from build123d import *

# Parameters (mm, degrees)
BOSS_EXTRUDE1_DEPTH                           = 10
CBORE_FOR_M3_HEX_HEAD_MACHINE_SCREW3_AT_COUNT = 2
CBORE_FOR_M3_HEX_HEAD_MACHINE_SCREW3_AT_PITCH = 31.112698372
CBORE_FOR_M3_HEX_HEAD_MACHINE_SCREW3_2_COUNT  = 2
CBORE_FOR_M3_HEX_HEAD_MACHINE_SCREW3_2_PITCH  = 44
CUT_EXTRUDE1_START                            = -10
CUT_EXTRUDE1_DEPTH                            = 10


with BuildPart() as part:
    # Sketch1 → Boss-Extrude1 (new body)
    with BuildSketch(Plane.XY):
        with BuildLine():
            Line((-2.236067977, -2), (-21, -2))
            Line((-21, -2), (-21, 2))
            Line((-21, 2), (-2.236067977, 2))
            ThreePointArc((-2.236067977, 2), (0, 3), (2.236067977, 2))
            Line((2.236067977, 2), (24.919871589, 2))
            ThreePointArc((24.919871589, 2), (-25, 0), (24.919871589, -2))
            Line((24.919871589, -2), (2.236067977, -2))
            ThreePointArc((2.236067977, -2), (0, -3), (-2.236067977, -2))
        make_face()
    extrude(amount=BOSS_EXTRUDE1_DEPTH)

    # Sketch6 → CBORE for M3 Hex Head Machine Screw2 (revolve, cut)
    with BuildSketch(Plane(origin=(19.919871589, 22, 5), x_dir=(0, 0, 1), z_dir=(1, 0, 0))):
        Polygon((0, 0), (0, 47), (1.7, 47), (1.7, 17.3), (4.2, 17.3), (4.2, 0.025), (4.225, 0), align=None)
    revolve(axis=Axis((19.919871589, 28.35, 5), (0, -1, 0)), mode=Mode.SUBTRACT)

    # Sketch8 → CBORE for M3 Hex Head Machine Screw3 (revolve, cut)
    with BuildSketch(Plane(origin=(-15.556349186, 15.556349186, 10), x_dir=(0, -1, 0), z_dir=(1, 0, 0))):
        Polygon((0, 0), (0, 10), (1.7, 10), (1.7, 2.3), (4.2, 2.3), (4.2, 0.025), (4.225, 0), align=None)
    cbore_for_m3_hex_head_machine_screw3 = revolve(axis=Axis((-15.556349186, 15.556349186, 16.35), (0, 0, -1)), mode=Mode.SUBTRACT)

    # CBORE for M3 Hex Head Machine Screw3 at: CBORE for M3 Hex Head Machine Screw3 ×2
    with Locations(*[(0, -i * CBORE_FOR_M3_HEX_HEAD_MACHINE_SCREW3_AT_PITCH, 0) for i in range(1, CBORE_FOR_M3_HEX_HEAD_MACHINE_SCREW3_AT_COUNT)]):
        add(cbore_for_m3_hex_head_machine_screw3, mode=Mode.SUBTRACT)

    # CBORE for M3 Hex Head Machine Screw3 2: CBORE for M3 Hex Head Machine Screw3 ×2
    with Locations(*[Vector(0.707106781, -0.707106781, 0) * (i * CBORE_FOR_M3_HEX_HEAD_MACHINE_SCREW3_2_PITCH) for i in range(1, CBORE_FOR_M3_HEX_HEAD_MACHINE_SCREW3_2_COUNT)]):
        add(cbore_for_m3_hex_head_machine_screw3, mode=Mode.SUBTRACT)

    # Sketch9 → Cut-Extrude1 (cut)
    with BuildSketch(Plane(origin=(0, 0, 0), x_dir=(-1, 0, 0), z_dir=(0, 0, -1)).offset(CUT_EXTRUDE1_START)):
        with BuildLine():
            ThreePointArc((-17.370952766, 13.5), (-19.8577472, 9.46941794), (-21.424285286, 5))
            Line((-21.424285286, 5), (21.424285286, 5))
            ThreePointArc((21.424285286, 5), (20.018217875, 9.125291947), (17.826515683, 12.892452777))
            ThreePointArc((17.826515683, 12.892452777), (15.142522709, 12.080899913), (12.724136619, 13.5))
            Line((12.724136619, 13.5), (-17.370952766, 13.5))
        make_face()
        with BuildLine():
            Line((21.424285286, -5), (-21.424285286, -5))
            ThreePointArc((-21.424285286, -5), (-20.018217875, -9.125291947), (-17.826515683, -12.892452777))
            ThreePointArc((-17.826515683, -12.892452777), (-15.142522709, -12.080899913), (-12.724136619, -13.5))
            Line((-12.724136619, -13.5), (12.724136619, -13.5))
            ThreePointArc((12.724136619, -13.5), (15.142522709, -12.080899913), (17.826515683, -12.892452777))
            ThreePointArc((17.826515683, -12.892452777), (20.018217875, -9.125291947), (21.424285286, -5))
        make_face()
        with BuildLine():
            ThreePointArc((12.892452777, 17.826515683), (-0.676730397, 21.989589263), (-13.964240044, 17))
            Line((-13.964240044, 17), (12.367952673, 17))
            ThreePointArc((12.367952673, 17), (12.601164732, 17.431685114), (12.892452777, 17.826515683))
        make_face()
        with BuildLine():
            ThreePointArc((-12.367952673, -17), (-12.601164732, -17.431685114), (-12.892452777, -17.826515683))
            ThreePointArc((-12.892452777, -17.826515683), (0, -22), (12.892452777, -17.826515683))
            ThreePointArc((12.892452777, -17.826515683), (12.601164732, -17.431685114), (12.367952673, -17))
            Line((12.367952673, -17), (-12.367952673, -17))
        make_face()
    extrude(amount=CUT_EXTRUDE1_DEPTH, mode=Mode.SUBTRACT)


solid = part.part
Part model, mm, in its own coordinate system. A direction names the side the tool comes from. Give positions to 0.01 mm unless a question says otherwise; leave off trailing zeros. Loops run counter-clockwise (first coordinate to the right, second up) from the corner with the lowest first, then second, coordinate; pieces in that order, holes last. Notation, with made-up numbers: (-11.75, -30) -> (21.25, -30) arc R14 cw to (21.25, -4) -> close; hole circle Ø2 at (54, -17). An arc over 180 degrees is marked (long way). Write each question's results on one line, items separated by ' | '. Start each with the question number.
Q1. Pin check, flat tips, straight feed: P1, Ø5.5, axis at x = -15.56, y = 15.56, coming from the +Z side; P2, Ø4, axis at y = -17.5, z = 2.5, coming from the +X side; P3, Ø3, axis at x = 4, z = 7, coming from the -Y side; P4, Ø5, axis at x = 0, y = -9.5, coming from the -Z side. Stop position of each tip, or through.
Q2. Band-saw the part on C-C on z = 2.5. Count the separate pieces of the cut face and the enclosed holes in it, plus the area to 3 significant figures.
Q3. Which spindle directions (+Z, -Z, +X, -X, +Y, -Y) get a long thin tool onto all of the face, cutting with end or side? Do faces 5 (the face through (11.37, -15.24, 8.85)), 6 (the face through (-13.684, 19.316, 8.853)), 7 (the face through (-21, 0, 5)). Say none if no direction does.
Q4. Band-saw the part on D-D on x = 0. List the corners of the cut face in (y, z), plus the area to 3 significant figures.
Q5. Pull direction Y, two halves, no side cores. Call faces 1 (the face through (0, 3, 5)), 2 (the face through (13.684, -19.316, 8.853)), 3 (the face through (18.234, 3.369, 4.779)), 4 (the face through (-19.294, 13.641, 8.853)): +Y half, -Y half, draft (parallel to the pull), parting line (faces both ways), or undercut.
Q6. Band-saw the part on B-B on y = 7. List the corners of the cut face in (x, z).
Q7. Wall check: L1, parallel to Y at x = 17.5, z = 7.75; L2, parallel to Y at x = 9, z = 5; L3, parallel to Y at x = 2.5, z = 9. Give the ranges that are in metal, low to high.
Q8. Band-saw the part on A-A on x = -5. List the corners of the cut face in (y, z).
Results are:
1) P1: stops at z = 7.7 | P2: stops at x = 19.62 | P3: stops at y = -24.87 | P4: passes through
2) separate pieces: 1 | enclosed holes: 6 | area: 861 mm²
3) face 5: +Z | face 6: +Z, -X | face 7: +Z, -Z, +X
4) outline: (-25, 0) -> (-22, 0) -> (-22, 10) -> (-25, 10) -> close; (-17, 0) -> (-13.5, 0) -> (-13.5, 10) -> (-17, 10) -> close; (-5, 0) -> (-3, 0) -> (-3, 10) -> (-5, 10) -> close; (3, 0) -> (5, 0) -> (5, 10) -> (3, 10) -> close; (13.5, 0) -> (17, 0) -> (17, 10) -> (13.5, 10) -> close; (22, 0) -> (25, 0) -> (25, 10) -> (22, 10) -> close | area: 170 mm²
5) face 1: undercut | face 2: undercut | face 3: draft | face 4: +Y half
6) outline: (-24, 0) -> (-20.86, 0) -> (-20.86, 10) -> (-24, 10) -> close; (20.86, 0) -> (24, 0) -> (24, 4) arc R4.2 cw to (20.86, 0.91) -> close; (20.86, 9.09) arc R4.2 cw to (24, 6) -> (24, 10) -> (20.86, 10) -> close
7) L1: y = -5 to -2, 2 to 4.7 | L2: y = -23.32 to -20.07, -17 to -13.5, -5 to -2, 2 to 5, 13.5 to 17, 20.07 to 23.32 | L3: y = -24.87 to -21.86, -17 to -13.5, -5 to -2, 2 to 5, 13.5 to 17, 21.86 to 24.87
8) outline: (-24.49, 0) -> (-21.42, 0) -> (-21.42, 10) -> (-24.49, 10) -> close; (-17, 0) -> (-13.5, 0) -> (-13.5, 10) -> (-17, 10) -> close; (-5, 0) -> (-2, 0) -> (-2, 10) -> (-5, 10) -> close; (2, 0) -> (5, 0) -> (5, 10) -> (2, 10) -> close; (13.5, 0) -> (17, 0) -> (17, 10) -> (13.5, 10) -> close; (21.42, 0) -> (24.49, 0) -> (24.49, 10) -> (21.42, 10) -> close
